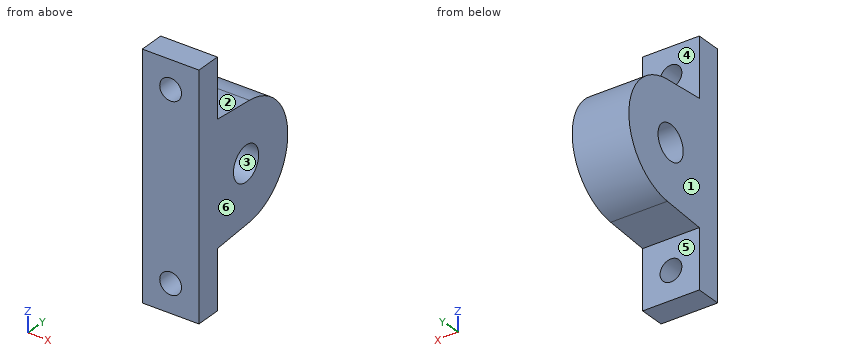
```python
from build123d import *

# Parameters (mm, degrees)
SKETCH1_R               = 4
BOSS_EXTRUDE1_DEPTH     = 13
CUT_EXTRUDE1_DEPTH      = 38.750758176
CUT_EXTRUDE1_DEPTH_BACK = 38.750758176
SKETCH2_R               = 2.5


with BuildPart() as part:
    # Sketch1 → Boss-Extrude1 (new body)
    with BuildSketch(Plane(origin=(0, 0, 0), x_dir=(0, 0, -1), z_dir=(1, 0, 0))):
        with BuildLine():
            Line((27.5, -14.95), (-27.5, -14.95))
            Line((-27.5, -14.95), (-27.5, -9.107766946))
            Line((-27.5, -9.107766946), (-14, -9.107766946))
            Line((-14, -9.107766946), (-13.209942251, 1.029526948))
            ThreePointArc((-13.209942251, 1.029526948), (0, 13.25), (13.209942251, 1.029526948))
            Line((13.209942251, 1.029526948), (14, -9.107766946))
            Line((14, -9.107766946), (27.5, -9.107766946))
            Line((27.5, -9.107766946), (27.5, -14.95))
        make_face()
        with Locations(Location((0, 0, 0), (0, 0, 180))):
            Circle(SKETCH1_R, mode=Mode.SUBTRACT)
    extrude(amount=BOSS_EXTRUDE1_DEPTH)

    # Sketch2 → Cut-Extrude1 (cut, two sides: drawn at the far end of the back side and taken through both)
    with BuildSketch(Plane(origin=(0, -9.107766946, 0), x_dir=(1, 0, 0), z_dir=(0, 1, 0)).offset(-CUT_EXTRUDE1_DEPTH_BACK)):
        with Locations(Location((6.5, 21, 0), (0, 0, 270))):
            Circle(SKETCH2_R)
        with Locations(Location((6.5, -21, 0), (0, 0, 90))):
            Circle(SKETCH2_R)
    extrude(amount=CUT_EXTRUDE1_DEPTH + CUT_EXTRUDE1_DEPTH_BACK, mode=Mode.SUBTRACT)


solid = part.part
```
Could you check a few things on this model? Use its own coordinates, in mm. Face numbers are marked on the shaded views. A direction names the side the tool comes from. Round coordinates to 2 decimals unless told otherwise and drop trailing zeros. Write each loop counter-clockwise with the first axis right and the second up, starting at its lowest first coordinate (ties: lowest second). Pieces come first, ordered by that corner, then holes.
(1) Suppose I cut it at B-B on z = -22.5. Write out the boundary of the cut face in (x, y).
Findings below:
outline: (0, -14.95) - (4.5, -14.95) - (4.5, -9.11) - (0, -9.11) - close; (8.5, -14.95) - (13, -14.95) - (13, -9.11) - (8.5, -9.11) - close
(2) Suppose I cut it at D-D on x = 12. Write out the boundary of the cut face in (y, z), and give its area (3 significant figures).
Findings below:
outline: (-14.95, -27.5) - (-9.11, -27.5) - (-9.11, -14) - (1.03, -13.21) arc R13.25 ccw to (1.03, 13.21) - (-9.11, 14) - (-9.11, 27.5) - (-14.95, 27.5) - close; hole circle Ø8 at (0, 0)
area: 795 mm2
(3) Which directions (+Z, -Z, +X, -X, +Y, -Y) give clear straight access to the entire face, cutting with the end or side of a thin tool? Please do the marked faces 4, 5 and 6.
Findings below:
face 4: +Z, +X, -X, +Y
face 5: -Z, +X, -X, +Y
face 6: +Z, -Z, +X, +Y, -Y
(4) Suppose I cut it at C-C on y = 0. Write out the boundary of the cut face in (x, z).
Findings below:
outline: (0, -13.29) - (13, -13.29) - (13, -4) - (0, -4) - close; (0, 4) - (13, 4) - (13, 13.29) - (0, 13.29) - close
(5) Suppose I cut it at A-A on x = 5.25. Write out the boundary of the cut face in (y, z), and give its area (3 significant figures).
Findings below:
outline: (-14.95, -27.5) - (-9.11, -27.5) - (-9.11, -23.17) - (-14.95, -23.17) - close; (-14.95, -18.83) - (-9.11, -18.83) - (-9.11, -14) - (1.03, -13.21) arc R13.25 ccw to (1.03, 13.21) - (-9.11, 14) - (-9.11, 18.83) - (-14.95, 18.83) - close; (-14.95, 23.17) - (-9.11, 23.17) - (-9.11, 27.5) - (-14.95, 27.5) - close; hole circle Ø8 at (0, 0)
area: 745 mm2
(6) For pin 1 (3 mm diameter, centred on x = 6, y = 9.5, fed in from -Z); pin 2 (1.5 mm diameter, centred on x = 8.5, z = -15, fed in from +Y); pin 3 (6 mm diameter, centred on x = 1.5, y = -5.5, fed in from -Z), each with a flat end and sliding along its axis, tell me the tip position at first contact or that it passes through.
Findings below:
pin 1: stops at z = -10.56
pin 2: stops at y = -9.11
pin 3: stops at z = -13.95
(7) Thinking about a two-plate mould opening in Y: for the marked faces 1, 2 and 3, which applies, +Y half, -Y half, draft (parallel to the pull), parting line (faces both ways), or undercut?
Findings below:
face 1: draft
face 2: +Y half
face 3: undercut
(8) If I drill on probe 1 along X at (y, z) = (-11.4, 21); probe 2 along Y at (x, z) = (3.25, -15.5); probe 3 along Z at (x, y) = (9.5, 1.25), over which ranges is the centre line in solid material (lowest first)?
Findings below:
probe 1: x = 0 to 4, 9 to 13
probe 2: y = -14.95 to -9.11
probe 3: z = -13.19 to -3.8, 3.8 to 13.19
